Here's how the part is built. I have some questions about the finished solid (model axes, mm). A direction names the side the tool comes from. Round coordinates to 2 decimals unless told otherwise and drop trailing zeros. Write each loop counter-clockwise with the first axis right and the second up, starting at its lowest first coordinate (ties: lowest second). Pieces come first, ordered by that corner, then holes. Notation, with made-up numbers: (41, 23.25) - (67, 23.25) arc R27 cw to (67, 44.25) - close; hole circle Ø11 at (-13.75, 75). An arc over 180 degrees is marked (long way). One line per item, written item: value. Start each with the question number.
Item 1: Imagine slicing it at A-A, the plane y = 5. Please give me the cut outline in (x, z), then the cut area to 3 significant figures.
Item 2: Imagine slicing it at B-B, the plane z = 0. Please give me the cut outline in (x, y), then the cut area to 3 significant figures.
Item 3: For P1, Ø19, axis at x = -30, z = 30, coming from the +Y side; P2, Ø3, axis at x = 24.5, y = 21.5, coming from the -Z side; P3, Ø4, axis at y = 15, z = -6, coming from the +X side; P4, Ø15.5, axis at x = -30, z = -30, coming from the -Y side, each with a flat end and sliding along its axis, tell me the tip position at first contact or that it passes through.
Item 4: Imagine slicing it at C-C, the plane y = 14. Please give me the cut outline in (x, z).
Item 5: Thinking about a two-plate mould opening in Z: for faces 1 (the face through (26, 47, 0)), 2 (the face through (-35.857, 5.916, 28.699)), 3 (the face through (-40.49, 5.92, -40.72)), which applies, released by +Z, released by -Z, zero draft, split by the parting line, or undercut?
Item 6: If I drill on line 1 (Z direction, x = 0, y = 16); line 2 (Y direction, x = 54.5, z = -1.5); line 3 (Z direction, x = 24, y = 37), over which ranges is the centre line in solid material (lowest first)?
Item 7: For faces 4 (the face through (3, 51, 6)), 5 (the face through (25, 24, -10)), 6 (the face through (18.54, 42.95, 0.78)), 7 (the face through (25, 25, 10)), which set-ups out of +Z, -Z, +X, -X, +Y, -Y let a thin tool reach every point of the face, with its end or its side?
Item 8: Imagine slicing it at D-D, the plane x = 70. Please give me the cut outline in (y, z).
```python
from build123d import *

# Parameters (mm, degrees)
SKETCH1_R           = 6
SKETCH1_R_2         = 7.5
BOSS_EXTRUDE1_DEPTH = 12
SKETCH2_R           = 22.5
BOSS_EXTRUDE2_DEPTH = 48
HOLE1_D             = 12
HOLE1_DEPTH         = 100
HOLE1_CBORE_D       = 28
HOLE1_CBORE_DEPTH   = 9
BOSS_EXTRUDE5_START = 15
BOSS_EXTRUDE5_DEPTH = 15
HOLE2_REACH         = 108.066
HOLE2_BORE_R        = 6


with BuildPart() as part:
    # Sketch1 → Boss-Extrude1 (new body)
    with BuildSketch(Plane(origin=(0, 0, 0), x_dir=(1, 0, 0), z_dir=(0, 1, 0))):
        with BuildLine():
            Line((-45, 30), (-45, -30))
            ThreePointArc((-45, -30), (-40.606601718, -40.606601718), (-30, -45))
            Line((-30, -45), (30, -45))
            Line((30, -45), (79.965290711, -19.613591743))
            ThreePointArc((79.965290711, -19.613591743), (91.923986167, 1.827246717), (76.580979422, 20.992634657))
            Line((76.580979422, 20.992634657), (0, 45))
            Line((0, 45), (-30, 45))
            ThreePointArc((-30, 45), (-40.606601718, 40.606601718), (-45, 30))
        make_face()
        with Locations(Location((-30, 30, 0), (0, 0, 270))):
            Circle(SKETCH1_R, mode=Mode.SUBTRACT)
        with Locations(Location((-30, -30, 0), (0, 0, 270))):
            Circle(SKETCH1_R, mode=Mode.SUBTRACT)
        with Locations(Location((70, 0, 0), (0, 0, 270))):
            Circle(SKETCH1_R_2, mode=Mode.SUBTRACT)
    extrude(amount=BOSS_EXTRUDE1_DEPTH)

    # Sketch2 → Boss-Extrude2 (add)
    with BuildSketch(Plane(origin=(0, 12, 0), x_dir=(1, 0, 0), z_dir=(0, 1, 0))):
        with Locations(Location((0, 0, 0), (0, 0, 270))):
            Circle(SKETCH2_R)
    extrude(amount=BOSS_EXTRUDE2_DEPTH)

    # Hole1
    with Locations(Plane(origin=(0, 60, 0), x_dir=(1, 0, 0), z_dir=(0, 1, 0))):
        with Locations((0, 0)):
            CounterBoreHole(HOLE1_D / 2, HOLE1_CBORE_D / 2, HOLE1_CBORE_DEPTH, depth=HOLE1_DEPTH)

    # Sketch5 → Boss-Extrude5 (add)
    with BuildSketch(Plane(origin=(0, 0, 0), x_dir=(0, 0, -1), z_dir=(1, 0, 0)).offset(BOSS_EXTRUDE5_START)):
        with BuildLine():
            Line((-10, 37), (-10, 0))
            Line((-10, 0), (10, 0))
            Line((10, 0), (10, 37))
            ThreePointArc((10, 37), (0, 47), (-10, 37))
        make_face()
    extrude(amount=BOSS_EXTRUDE5_DEPTH)

    # Hole2 bore → Hole2 (cut, up to next)
    with BuildSketch(Plane(origin=(30, 0, 0), x_dir=(0, 0, -1), z_dir=(1, 0, 0)), mode=Mode.PRIVATE) as hole2_sk1:
        with Locations((0, 37)):
            Circle(HOLE2_BORE_R)
    hole2_tool1 = extrude(hole2_sk1.sketch, amount=-HOLE2_REACH, mode=Mode.PRIVATE) & part.part
    add(hole2_tool1.solids().sort_by_distance((30, 37, 0))[0], mode=Mode.SUBTRACT)


solid = part.part
```
Values follow:
1. outline: (-45, -30) arc R15 ccw to (-30, -45) - (0, -45) - (76.58, -20.99) arc R22 ccw to (79.97, 19.61) - (30, 45) - (-30, 45) arc R15 ccw to (-45, 30) - close; hole circle Ø12 at (-30, -30); hole circle Ø12 at (-30, 30); hole circle Ø12 at (0, 0); hole circle Ø15 at (70, 0)
1. area: 9,330 mm^2
2. outline: (-45, 0) - (-6, 0) - (-6, 51) - (-14, 51) - (-14, 60) - (-22.5, 60) - (-22.5, 12) - (-45, 12) - close; (6, 0) - (62.5, 0) - (62.5, 12) - (30, 12) - (30, 31) - (6, 31) - close; (6, 43) - (30, 43) - (30, 47) - (22.5, 47) - (22.5, 60) - (14, 60) - (14, 51) - (6, 51) - close; (77.5, 0) - (92, 0) - (92, 12) - (77.5, 12) - close
2. area: 2,730 mm^2
3. P1: stops at y = 12
3. P2: stops at z = -10
3. P3: stops at x = 30
3. P4: stops at y = 0
4. outline: (20.16, -10) - (30, -10) - (30, 10) - (20.16, 10) arc R22.5 ccw (long way) to start; hole circle Ø12 at (0, 0)
5. face 1: split by the parting line
5. face 2: undercut
5. face 3: released by -Z
6. line 1: z = -22.5 to -6, 6 to 22.5
6. line 2: y = 0 to 12
6. line 3: z = -10 to -6, 6 to 10
7. face 4: +Y
7. face 5: -Z, +X, +Y
7. face 6: +X
7. face 7: +Z, +X, +Y
8. outline: (0, -23.06) - (12, -23.06) - (12, -7.5) - (0, -7.5) - close; (0, 7.5) - (12, 7.5) - (12, 24.68) - (0, 24.68) - close
